```python
from build123d import *

# Parameters (mm, degrees)
ESQUISSE2_W             = 370.3
ESQUISSE2_H             = 330.3
BOSS_EXTRU_1_DEPTH      = 8
CONG_1_R                = 10
CHANFREIN1_SIZE         = 50
ESQUISSE4_R             = 4
ENL_V_MAT_EXTRU_1_DEPTH = 10
ESQUISSE5_R             = 7
ENL_V_MAT_EXTRU_2_DEPTH = 5
ESQUISSE6_R             = 4.1
ENL_V_MAT_EXTRU_3_DEPTH = 10


with BuildPart() as part:
    # Esquisse2 → Boss.-Extru.1 (new body)
    with BuildSketch(Plane.XY):
        with Locations((0, 191)):
            Rectangle(ESQUISSE2_W, ESQUISSE2_H)
    extrude(amount=BOSS_EXTRU_1_DEPTH)

    # Congé1
    cong_1_edges = [part.edges().sort_by_distance(p)[0] for p in [
        (-185.15, 356.15, 4),
        (185.15, 356.15, 4),
    ]]
    fillet(cong_1_edges, radius=CONG_1_R)

    # Chanfrein1
    chanfrein1_edges = [part.edges().sort_by_distance(p)[0] for p in [
        (185.15, 25.85, 4),
        (-185.15, 25.85, 4),
    ]]
    chamfer(chanfrein1_edges, length=CHANFREIN1_SIZE)

    # Esquisse4 → Enlèv. mat.-Extru.1 (cut)
    with BuildSketch(Plane.XY.offset(8)):
        with Locations((30, 170.289321881)):
            Circle(ESQUISSE4_R)
        with Locations(Location((-30, 170.289321881, 0), (0, 0, 180))):
            Circle(ESQUISSE4_R)
        with Locations((-33.142135624, 266.568542495)):
            Circle(ESQUISSE4_R)
        with Locations(Location((-75.568542495, 224.142135624, 0), (0, 0, 180))):
            Circle(ESQUISSE4_R)
        with Locations((33.142135624, 266.568542495)):
            Circle(ESQUISSE4_R)
        with Locations(Location((75.568542495, 224.142135624, 0), (0, 0, 180))):
            Circle(ESQUISSE4_R)
        with Locations((30, 40.85)):
            Circle(ESQUISSE4_R)
        with Locations(Location((-30, 40.85, 0), (0, 0, 180))):
            Circle(ESQUISSE4_R)
        with Locations((-100.652525317, 341.15)):
            Circle(ESQUISSE4_R)
        with Locations(Location((-150.15, 291.652525317, 0), (0, 0, 180))):
            Circle(ESQUISSE4_R)
        with Locations(Location((100.652525317, 341.15, 0), (0, 0, 180))):
            Circle(ESQUISSE4_R)
        with Locations((150.15, 291.652525317)):
            Circle(ESQUISSE4_R)
    extrude(amount=-ENL_V_MAT_EXTRU_1_DEPTH, mode=Mode.SUBTRACT)

    # Esquisse5 → Enlèv. mat.-Extru.2 (cut)
    with BuildSketch(Plane.XY.offset(8)):
        with Locations((30, 40.85)):
            Circle(ESQUISSE5_R)
        with Locations((-30, 40.85)):
            Circle(ESQUISSE5_R)
        with Locations((30, 170.289321881)):
            Circle(ESQUISSE5_R)
        with Locations((-30, 170.289321881)):
            Circle(ESQUISSE5_R)
        with Locations((75.568542495, 224.142135624)):
            Circle(ESQUISSE5_R)
        with Locations((33.142135624, 266.568542495)):
            Circle(ESQUISSE5_R)
        with Locations((150.15, 291.652525317)):
            Circle(ESQUISSE5_R)
        with Locations((100.652525317, 341.15)):
            Circle(ESQUISSE5_R)
        with Locations((-33.142135624, 266.568542495)):
            Circle(ESQUISSE5_R)
        with Locations((-75.568542495, 224.142135624)):
            Circle(ESQUISSE5_R)
        with Locations((-150.15, 291.652525317)):
            Circle(ESQUISSE5_R)
        with Locations((-100.652525317, 341.15)):
            Circle(ESQUISSE5_R)
    extrude(amount=-ENL_V_MAT_EXTRU_2_DEPTH, mode=Mode.SUBTRACT)

    # Esquisse6 → Enlèv. mat.-Extru.3 (cut)
    with BuildSketch(Plane.XY.offset(8)):
        with Locations((165.15, 75.85)):
            Circle(ESQUISSE6_R)
        with Locations((110.15, 75.85)):
            Circle(ESQUISSE6_R)
        with Locations((55.15, 75.85)):
            Circle(ESQUISSE6_R)
        with Locations((0.15, 75.85)):
            Circle(ESQUISSE6_R)
        with Locations((-54.85, 75.85)):
            Circle(ESQUISSE6_R)
        with Locations((-109.85, 75.85)):
            Circle(ESQUISSE6_R)
        with Locations((-164.85, 75.85)):
            Circle(ESQUISSE6_R)
        with Locations((110.15, 130.85)):
            Circle(ESQUISSE6_R)
        with Locations((55.15, 130.85)):
            Circle(ESQUISSE6_R)
        with Locations((0.15, 130.85)):
            Circle(ESQUISSE6_R)
        with Locations((-54.85, 130.85)):
            Circle(ESQUISSE6_R)
        with Locations((-109.85, 130.85)):
            Circle(ESQUISSE6_R)
        with Locations((-164.85, 130.85)):
            Circle(ESQUISSE6_R)
        with Locations((110.15, 185.85)):
            Circle(ESQUISSE6_R)
        with Locations((55.15, 185.85)):
            Circle(ESQUISSE6_R)
        with Locations((0.15, 185.85)):
            Circle(ESQUISSE6_R)
        with Locations((-54.85, 185.85)):
            Circle(ESQUISSE6_R)
        with Locations((-109.85, 185.85)):
            Circle(ESQUISSE6_R)
        with Locations((-164.85, 185.85)):
            Circle(ESQUISSE6_R)
        with Locations((110.15, 240.85)):
            Circle(ESQUISSE6_R)
        with Locations((55.15, 240.85)):
            Circle(ESQUISSE6_R)
        with Locations((0.15, 240.85)):
            Circle(ESQUISSE6_R)
        with Locations((-54.85, 240.85)):
            Circle(ESQUISSE6_R)
        with Locations((-109.85, 240.85)):
            Circle(ESQUISSE6_R)
        with Locations((-164.85, 240.85)):
            Circle(ESQUISSE6_R)
        with Locations((110.15, 295.85)):
            Circle(ESQUISSE6_R)
        with Locations((55.15, 295.85)):
            Circle(ESQUISSE6_R)
        with Locations((0.15, 295.85)):
            Circle(ESQUISSE6_R)
        with Locations((-54.85, 295.85)):
            Circle(ESQUISSE6_R)
        with Locations((-109.85, 295.85)):
            Circle(ESQUISSE6_R)
        with Locations((-164.85, 295.85)):
            Circle(ESQUISSE6_R)
        with Locations((110.15, 350.85)):
            Circle(ESQUISSE6_R)
        with Locations((55.15, 350.85)):
            Circle(ESQUISSE6_R)
        with Locations((0.15, 350.85)):
            Circle(ESQUISSE6_R)
        with Locations((-54.85, 350.85)):
            Circle(ESQUISSE6_R)
        with Locations((-109.85, 350.85)):
            Circle(ESQUISSE6_R)
        with Locations((-164.85, 350.85)):
            Circle(ESQUISSE6_R)
        with Locations((165.15, 130.85)):
            Circle(ESQUISSE6_R)
        with Locations((165.15, 185.85)):
            Circle(ESQUISSE6_R)
        with Locations((165.15, 240.85)):
            Circle(ESQUISSE6_R)
        with Locations((165.15, 295.85)):
            Circle(ESQUISSE6_R)
        with Locations((165.15, 350.85)):
            Circle(ESQUISSE6_R)
        with Locations((110.15, 33.85)):
            Circle(ESQUISSE6_R)
        with Locations((55.15, 33.85)):
            Circle(ESQUISSE6_R)
        with Locations((0.15, 33.85)):
            Circle(ESQUISSE6_R)
        with Locations((-54.85, 33.85)):
            Circle(ESQUISSE6_R)
        with Locations((-109.85, 33.85)):
            Circle(ESQUISSE6_R)
    extrude(amount=-ENL_V_MAT_EXTRU_3_DEPTH, mode=Mode.SUBTRACT)


solid = part.part
```
Here's how the part is built. I have some questions about the finished solid (model axes, mm). A direction names the side the tool comes from. Give positions to 0.01 mm unless a question says otherwise; leave off trailing zeros.
(1) Thinking about a two-plate mould opening in Y: for faces 1 (the face through (-0.739, 346.847, 4.056)), 2 (the face through (-3, 193, 0)), which applies, pulls with the +Y half, pulls with the -Y half, needs draft (parallel to the pull), parting line crosses it, or undercut?
Output values:
face 1: undercut
face 2: needs draft
(2) On a 3-axis mill with a long thin cutter (end or side, diameter ignored), from which of +Z, -Z, +X, -X, +Y, -Y can I reach the whole of each face in a straight line? I mean faces 3 (the face through (57.04, 127.21, 4.06)), 4 (the face through (33, 37.8, 3)). Say none if no direction works.
Output values:
face 3: +Z, -Z
face 4: +Z
(3) If I drill on L1, parallel to X at y = 341.15, z = 0.85; L2, parallel to X at y = 223, z = 5.25; L3, parallel to X at y = 66.5, z = 2.25, over which ranges is the centre line in solid material (lowest first)?
Output values:
L1: x = -185.15 to -104.65, -96.65 to 96.65, 104.65 to 185.15
L2: x = -185.15 to -82.47, -68.66 to 68.66, 82.47 to 185.15
L3: x = -175.8 to 175.8
(4) Will these pins go through, and if not, where does the flat tip stop? pin 1 (6 mm diameter, centred on x = 35.5, y = 179, fed in from -Z); pin 2 (10.5 mm diameter, centred on x = -150.15, y = 291.65, fed in from +Z).
Output values:
pin 1: stops at z = 0
pin 2: stops at z = 3
(5) Imagine slicing it at A-A, the plane x = 55.15. Count the separate pieces of the cut face and the enclosed holes in it, and give its area (3 significant figures).
Output values:
separate pieces: 8
enclosed holes: 0
area: 2,180 mm2
